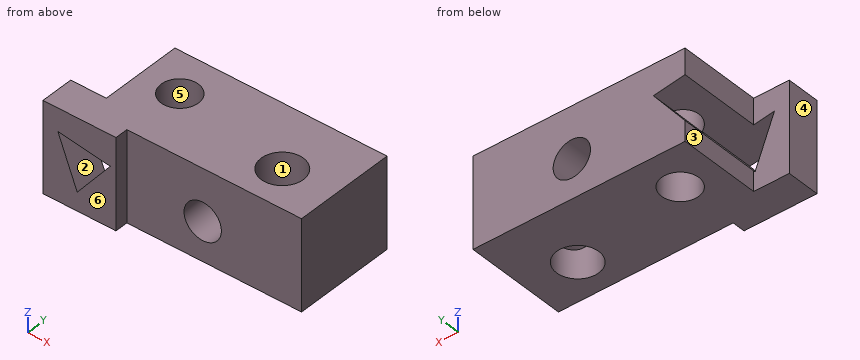
```python
from build123d import *

# Parameters (mm, degrees)
F0_R     = 17.76649
F0_R_2   = 15.679579
F1_DEPTH = 76.2
F3_DEPTH = 112.522
F4_R     = 15.719136
F5_DEPTH = 182.626
F6_R     = 16.325262
F6_R_2   = 3.503895
F7_DEPTH = 86.106


with BuildPart() as f1:
    # F0 (on Top) → F1 (new body)
    with BuildSketch(Plane.XY):
        Polygon((105.979137, 26.87672), (-72.61806, 26.87672), (-72.61806, -42.346146), (-102.592185, -42.346146), (-102.592185, -70.317619), (-41.133739, -70.317619), (-41.133739, -59.36873), (105.979137, -59.36873), align=None)
        with Locations((62.618658, -26.834318)):
            Circle(F0_R, mode=Mode.SUBTRACT)
        with Locations((-39.288443, -8.131367)):
            Circle(F0_R_2, mode=Mode.SUBTRACT)
    extrude(amount=-F1_DEPTH)

    # F2 (on face) → F3 (cut)
    with BuildSketch(Plane.XZ.offset(70.317619)):
        Polygon((-73.776924, -60.745504), (-45.90854, -25.806386), (-90.100896, -19.141217), align=None)
    extrude(amount=-F3_DEPTH, mode=Mode.SUBTRACT)

    # F4 (on face) → F5 (cut)
    with BuildSketch(Plane(origin=(0, 26.87672, 0), x_dir=(-1, 0, 0), z_dir=(0, 1, 0))):
        with Locations((-22.761121, -43.327287)):
            Circle(F4_R)
    extrude(amount=-F5_DEPTH, mode=Mode.SUBTRACT)

    # F6 (on face) → F7 (join)
    with BuildSketch(Plane(origin=(0, 26.87672, 0), x_dir=(-1, 0, 0), z_dir=(0, 1, 0))):
        with Locations((-78.335434, -36.600552)):
            Circle(F6_R)
        with Locations((-78.335434, -36.600552)):
            Circle(F6_R_2, mode=Mode.SUBTRACT)
    extrude(amount=-F7_DEPTH)


solid = f1.part
```
CAD build for the part. Positions are in the model's coordinates, mm. Face numbers are marked on the shaded views. A direction names the side the tool comes from. Round coordinates to 2 decimals unless told otherwise and drop trailing zeros. Order: outer loops, then holes, each group sorted by start corner. A loop starts at its lowest first (then second) coordinate and runs counter-clockwise, first axis right, second up. Notation, with made-up numbers: (-8, 23) - (8, 23) arc R19 ccw to (8, 58) - close; hole circle Ø10 at (86, -4.75). An arc over 180 degrees is marked (long way). Use CSV: the item, a comma, the result in double quotes. Start each with the question number.
1) Two-plate mould, pull along X, no slides. Class the marked faces 4, 5 and 6: pulls with the +X half, pulls with the -X half, needs draft (parallel to the pull), parting line crosses it, or undercut.
2) Tool access for the marked faces 1, 2 and 3: list every direction of +Z, -Z, +X, -X, +Y, -Y with a clear straight run to the whole face (end or side of a thin tool).
3) Saw through at A-A (y = -33.5). List the corners of the cut face in (x, z), and give its area (3 significant figures).
4) Saw through at D-D (x = -35). List the corners of the cut face in (y, z).
5) Saw through at C-C (z = -13.5). List the corners of the cut face in (x, y).
6) Saw through at B-B (y = -19). List the corners of the cut face in (x, z), and give its area (3 significant figures).
7) Pin check, flat tips, straight feed: pin 1 Ø4 at (x, z) = (78.34, -36.6) entering from -Y; pin 2 Ø1.5 at (x, y) = (-17, -20) entering from +Z; pin 3 Ø19 at (x, y) = (-39.29, -8.13) entering from +Z; pin 4 Ø17.5 at (y, z) = (-6.5, -12.5) entering from -X. Stop position of each tip, or through.
8) Wall check: L1, parallel to X at y = -11, z = -15; L2, parallel to X at y = -12, z = -68; L3, parallel to Y at x = 95, z = -5.5. Give the ranges that are in metal, low to high. Write a range as [from, to].
Values follow:
1,face 4,"pulls with the -X half"
1,face 5,"undercut"
1,face 6,"needs draft"
2,face 1,"none"
2,face 2,"+Y, -Y"
2,face 3,"+Z, -Z, -X, +Y"
3,outline,"(-72.62, -76.2) - (46.15, -76.2) - (46.15, 0) - (-72.62, 0) - (-72.62, -21.78) - (-45.91, -25.81) - (-72.62, -59.29) - close; (79.09, -76.2) - (105.98, -76.2) - (105.98, 0) - (79.09, 0) - (79.09, -20.29) arc R16.33 ccw (long way) to (79.09, -52.91) - close; hole circle Ø31.44 at (22.76, -43.33); hole (79.09, -40.02) - (79.09, -33.18) arc R3.5 ccw (long way) to start"
3,area,"10,200 mm2"
4,outline,"(-59.37, -76.2) - (-23.21, -76.2) - (-23.21, 0) - (-59.37, 0) - close; (6.95, -76.2) - (26.88, -76.2) - (26.88, 0) - (6.95, 0) - close"
5,outline,"(-102.59, -70.32) - (-41.13, -70.32) - (-41.13, -59.37) - (105.98, -59.37) - (105.98, 26.88) - (-72.62, 26.88) - (-72.62, -42.35) - (-102.59, -42.35) - close; hole circle Ø31.36 at (-39.29, -8.13); hole circle Ø35.53 at (62.62, -26.83)"
6,outline,"(-72.62, -76.2) - (-50.59, -76.2) - (-50.59, -31.68) - (-72.62, -59.29) - close; (-72.62, -21.78) - (-50.59, -25.1) - (-50.59, 0) - (-72.62, 0) - close; (-27.99, -76.2) - (46.67, -76.2) - (46.67, 0) - (-27.99, 0) - close; (78.56, -76.2) - (105.98, -76.2) - (105.98, 0) - (78.56, 0) - (78.56, -20.28) arc R16.33 ccw (long way) to (78.56, -52.92) - close; hole circle Ø31.44 at (22.76, -43.33); hole (78.56, -40.1) - (78.56, -33.1) arc R3.5 ccw (long way) to start"
6,area,"8,600 mm2"
7,pin 1,"stops at y = -59.37"
7,pin 2,"stops at z = 0"
7,pin 3,"passes through"
7,pin 4,"stops at x = -72.62"
8,L1,"x = [-72.62, -54.7], [-23.87, 54.56], [70.68, 105.98]"
8,L2,"x = [-72.62, -54.48], [-24.09, 52.84], [72.4, 105.98]"
8,L3,"y = [-59.37, 26.88]"
